```python
from build123d import *

# Parameters (mm, degrees)
BOSS_EXTRUDE2_DEPTH = 12.2
CUT_EXTRUDE1_DEPTH  = 30


with BuildPart() as part:
    # Sketch1 → Boss-Extrude2 (new body)
    with BuildSketch(Plane(origin=(0, 0, 0), x_dir=(1, 0, 0), z_dir=(0, 1, 0))):
        Polygon((150, 125), (-150, 125), (-150, 65), (-20, 65), (-20, -65), (-150, -65), (-150, -125), (150, -125), align=None)
    extrude(amount=BOSS_EXTRUDE2_DEPTH)

    # Sketch2 → Cut-Extrude1 (cut)
    with BuildSketch(Plane(origin=(0, 12.2, 0), x_dir=(1, 0, 0), z_dir=(0, 1, 0))):
        with BuildLine():
            Line((15.884395788, 39.654803454), (15.884395788, -39.654803454))
            ThreePointArc((15.884395788, -39.654803454), (11.884395788, -43.654803454), (7.884395788, -39.654803454))
            Line((7.884395788, -39.654803454), (7.884395788, 39.654803454))
            ThreePointArc((7.884395788, 39.654803454), (11.884395788, 43.654803454), (15.884395788, 39.654803454))
        make_face()
    extrude(amount=-CUT_EXTRUDE1_DEPTH, mode=Mode.SUBTRACT)


solid = part.part
```
The listing builds one solid part. Answer for the finished solid, in the listing's coordinates (mm). A direction names the side the tool comes from. Round coordinates to 2 decimals unless told otherwise and drop trailing zeros. Loops run counter-clockwise (first coordinate to the right, second up) from the corner with the lowest first, then second, coordinate; pieces in that order, holes last.
1) Consider line 1 (Z direction, x = -101, y = 8.25); line 2 (X direction, y = 10, z = 8.5); line 3 (X direction, y = 4.5, z = 49.5). Determine where each line is inside the solid, lowest interval first.
Outcome:
line 1: z = -125 to -65, 65 to 125
line 2: x = -20 to 7.88, 15.88 to 150
line 3: x = -20 to 150
2) A cutting plane is placed at A-A on x = -65.5. Determine the outline of the cut face in (y, z), plus the area to 3 significant figures.
Outcome:
outline: (0, -125) - (12.2, -125) - (12.2, -65) - (0, -65) - close; (0, 65) - (12.2, 65) - (12.2, 125) - (0, 125) - close
area: 1,460 mm2
3) For faces 1 (the face through (-84, 6, 65)), 2 (the face through (11.796, 6.185, -43.654)), 3 (the face through (31, 0, -2)), determine the directions among +Z, -Z, +X, -X, +Y, -Y from which every point of the face is accessible in a straight line to the end or side of a thin tool.
Outcome:
face 1: -X, +Y, -Y
face 2: +Y, -Y
face 3: +Z, -Z, +X, -X, -Y
4) A cutting plane is placed at C-C on y = 9. Determine the outline of the cut face in (x, z), plus the area to 3 significant figures.
Outcome:
outline: (-150, -125) - (150, -125) - (150, 125) - (-150, 125) - (-150, 65) - (-20, 65) - (-20, -65) - (-150, -65) - close; hole (7.88, -39.65) arc R4 ccw to (15.88, -39.65) - (15.88, 39.65) arc R4 ccw to (7.88, 39.65) - close
area: 57,400 mm2
5) A cutting plane is placed at D-D on z = -61. Determine the outline of the cut face in (x, y).
Outcome:
outline: (-20, 0) - (150, 0) - (150, 12.2) - (-20, 12.2) - close
6) A cutting plane is placed at B-B on z = 21. Determine the outline of the cut face in (x, y).
Outcome:
outline: (-20, 0) - (7.88, 0) - (7.88, 12.2) - (-20, 12.2) - close; (15.88, 0) - (150, 0) - (150, 12.2) - (15.88, 12.2) - close
7) Given P1, Ø6, axis at y = 7.5, z = -28.5, coming from the -X side, flat-ended and moving along its own axis, determine where the tip first touches the part or whether it passes through.
Outcome:
P1: stops at x = -20
